Autodesk Inventor part; units mm, degrees
ref_plane "YZ Plane" through (0, 0, 0) normal (1, 0, 0) x (0, 1, 0)
ref_plane "XZ Plane" through (0, 0, 0) normal (0, 1, 0) x (-1, 0, 0)
ref_plane "XY Plane" through (0, 0, 0) normal (0, 0, 1) x (1, 0, 0)
sketch "スケッチ1" plane through (0, 0, 0) normal (0, 1, 0) x (-1, 0, 0)
  line L0 (0, 0) -> (80, 0)
  line L1 (80, 0) -> (80, -142)
  line L2 (80, -142) -> (0, -142)
  line L3 (0, -142) -> (0, 0)
  dimension "d0" = 80
  dimension "d1" = 142
extrude "押し出し1" add sketch "スケッチ1" along normal blind 3.3
hole "穴1" at (-75.5, 3.3, -4.5) direction (0, -1, 0) diameter 3.4 end through all
hole "穴2" at (-4.5, 3.3, -4.5) direction (0, -1, 0) diameter 3.4 end through all
hole "穴3" at (-4.5, 3.3, -137.5) direction (0, -1, 0) diameter 3.4 end through all
hole "穴4" at (-75.5, 3.3, -137.5) direction (0, -1, 0) diameter 3.4 end through all
hole "穴5" at (-49, 3.3, -137.75) direction (0, -1, 0) diameter 2.4 end through all
hole "穴6" at (-31, 3.3, -137.75) direction (0, -1, 0) diameter 2.4 end through all
hole "穴7" at (-31, 3.3, -4.25) direction (0, -1, 0) diameter 2.4 end through all
hole "穴8" at (-49, 3.3, -4.25) direction (0, -1, 0) diameter 2.4 end through all
hole "穴9" at (-7, 0, -71) direction (0, 1, 0) diameter 2.4 end through all
hole "穴10" at (-23, 0, -71) direction (0, 1, 0) diameter 2.4 end through all
properties part number "基本板" material "アルミニウム 5052"
Can you work these out from the model? Positions are in its coordinate system, mm. Give positions to 0.01 mm unless a question says otherwise; leave off trailing zeros. Loops run counter-clockwise (first coordinate to the right, second up) from the corner with the lowest first, then second, coordinate; pieces in that order, holes last. Notation, with made-up numbers: (48, 74) -> (85, 74) arc R29 cw to (85, 107) -> close; hole circle Ø3 at (-34, 30). An arc over 180 degrees is marked (long way). Write item = value, one per line.
1) Suppose I cut it at A-A on x = -75.5. Write out the boundary of the cut face in (y, z).
Check result:
outline = (0, -142) -> (3.3, -142) -> (3.3, -139.2) -> (0, -139.2) -> close; (0, -135.8) -> (3.3, -135.8) -> (3.3, -6.2) -> (0, -6.2) -> close; (0, -2.8) -> (3.3, -2.8) -> (3.3, 0) -> (0, 0) -> close
2) I need wall thicknesses on L1, parallel to Z at x = -49, y = 2.55; L2, parallel to Z at x = -4.5, y = 0.9; L3, parallel to X at y = 2.6, z = -4.5. Which ranges of each line are inside material? Lowest first, please. Write a range as from..to.
Check result:
L1 = -142..-138.95, -136.55..-5.45, -3.05..0
L2 = -142..-139.2, -135.8..-6.2, -2.8..0
L3 = -80..-77.2, -73.8..-50.17, -47.83..-32.17, -29.83..-6.2, -2.8..0
3) Thinking about a two-plate mould opening in Z: for faces 1 (the flat face through (-39, 0, -70)), 2 (the cylindrical face through (-3.85, 1.63, -135.93)), 3 (the flat face through (-41, 2, -142)), 4 (the flat face through (-39, 2, 0)), which applies, released by +Z, released by -Z, zero draft, split by the parting line, or undercut?
Check result:
face_1 = zero draft
face_2 = undercut
face_3 = released by -Z
face_4 = released by +Z
4) Will this pin go through, and if not, where does the flat tip stop? pin 1 (1.9 mm diameter, centred on x = -7, z = -71, fed in from +Y).
Check result:
pin_1 = through
